The listing builds one solid part. Answer for the finished solid, in the listing's coordinates (mm). A direction names the side the tool comes from. Give positions to 0.01 mm unless a question says otherwise; leave off trailing zeros. Write each loop counter-clockwise with the first axis right and the second up, starting at its lowest first coordinate (ties: lowest second). Pieces come first, ordered by that corner, then holes. Notation, with made-up numbers: (16.5, 17.25) - (60.5, 17.25) arc R7 cw to (60.5, 21.25) - close; hole circle Ø5 at (-18.5, 15). An arc over 180 degrees is marked (long way). One line per question, with ' | ' between items. Start each with the question number.
1. For faces 1 (the face through (0, 0, 0)), 2 (the face through (0, 0.9, 29)), 3 (the face through (0, -2, 29)), determine the directions among +Z, -Z, +X, -X, +Y, -Y from which every point of the face is accessible in a straight line to the end or side of a thin tool.
2. Find the intervals of material crossed by L1, parallel to X at y = 0.9, z = 9; L2, parallel to Z at x = -0.8, y = 2.65; L3, parallel to X at y = -1, z = 2.5, in increasing order. Write a range as from..to.
3. A cutting plane is placed at A-A (y = 0). Determine the outline of the cut face in (x, z), then the cut area to 3 significant figures.
4. A cutting plane is placed at C-C (z = 19.5). Determine the outline of the cut face in (x, y).
5. A cutting plane is placed at B-B (x = 0). Determine the outline of the cut face in (y, z), then the cut area to 3 significant figures.
6. Given P1, Ø1.6, axis at x = -0.5, z = 29, coming from the +Y side; P2, Ø1, axis at y = -1, z = 11, coming from the -X side; P3, Ø3, axis at y = 2.5, z = 14.5, coming from the +X side, each flat-ended and moving along its own axis, determine where each tip first touches the part or whether it passes through.
Autodesk Inventor part; units mm, degrees
ref_plane "YZ Plane" through (0, 0, 0) normal (1, 0, 0) x (0, 1, 0)
ref_plane "XZ Plane" through (0, 0, 0) normal (0, 1, 0) x (-1, 0, 0)
ref_plane "XY Plane" through (0, 0, 0) normal (0, 0, 1) x (1, 0, 0)
sketch "スケッチ1" plane through (0, 0, 0) normal (0, 0, 1) x (1, 0, 0)
  circle A0 centre (0, 0) radius 3
  dimension "d0" = 6
extrude "押し出し1" add sketch "スケッチ1" along normal blind 30
chamfer "面取り1" distance 0.5 angle 15 2 edges at (-3, 0, 0) (-3, 0, 30) measured on face at (2.9903, -0.2414, 20)
sketch "スケッチ2" plane through (0, 0, 30) normal (0, 0, 1) x (1, 0, 0)
  circle A0 centre (0, 0) radius 3
  circle A1 centre (0, 0) radius 2
  line L0 (-1.7861, 0.9) -> (1.7861, 0.9)
  dimension "d7" = 4
  dimension "d8" = 0.9
extrude "押し出し2" cut sketch "スケッチ2" against normal blind 2 contours A0 | L0 A1 picked at (-0.2398, 1.4933)
properties part number "平行ピンD6L30Dcut" material "ステンレス鋼"
Determined:
1) face 1: -Z, +X, -X, +Y, -Y | face 2: +Z, +X, -X, +Y | face 3: +Z
2) L1: -2.86..2.86 | L2: 0..28 | L3: -2.83..2.83
3) outline: (-3, 0.5) - (-2.87, 0) - (2.87, 0) - (3, 0.5) - (3, 28) - (2, 28) - (2, 30) - (-2, 30) - (-2, 28) - (-3, 28) - close | area: 176 mm2
4) outline: circle Ø6 at (0, 0)
5) outline: (-3, 0.5) - (-2.87, 0) - (2.87, 0) - (3, 0.5) - (3, 28) - (0.9, 28) - (0.9, 30) - (-2, 30) - (-2, 28) - (-3, 28) - close | area: 174 mm2
6) P1: y = 0.9 | P2: x = -2.96 | P3: x = 2.83
